Model file for the job. Use its own axes, mm. A direction names the side the tool comes from. Round coordinates to 2 decimals unless told otherwise and drop trailing zeros. Order: outer loops, then holes, each group sorted by start corner. A loop starts at its lowest first (then second) coordinate and runs counter-clockwise, first axis right, second up. Notation, with made-up numbers: (16.5, 23.5) -> (69.5, 23.5) arc R23 ccw to (69.5, 54.5) -> close; hole circle Ø9 at (25.5, 38.25). An arc over 180 degrees is marked (long way). Put each result on its own line as item: value. Start each with the question number.
Q1. Cut at C-C, the plane x = 27. List the corners of the cut face in (y, z) (3 decimals).
Q2. Flat gauge pins, fed straight in: P1, Ø10, axis at x = 20, y = 38.5, coming from the -Z side; P2, Ø7.5, axis at y = 7, z = -14, coming from the -X side; P3, Ø5, axis at x = 27, y = -4.5, coming from the +Z side (3 decimals). Where does each tip first touch, or does it go through?
Q3. Pull direction Z, two halves, no side cores. Call faces 1 (the face through (20, 8, -20)), 2 (the face through (21.035, 7.973, -10.515)), 3 (the face through (30, 68, -15)), 4 (the face through (13, 117, 15)): released by +Z, released by -Z, zero draft, split by the parting line, or undercut.
Q4. Cut at A-A, the plane y = 6.56. List the corners of the cut face in (x, z), and give its area (3 significant figures).
Q5. Cut at D-D, the plane z = -3.5. List the corners of the cut face in (x, y).
Q6. 3-axis set-ups, long thin cutter, end or side, ignore diameter. For faces 5 (the face through (25, -8, -8.025)), 6 (the face through (15, 44, -30)), 7 (the face through (10, 15, -4.95)): which of +Z, -Z, +X, -X, +Y, -Y reach the whole face in a straight line?
Q7. Cut at B-B, the plane z = -15. State how many separate pieces and enclosed holes the cut face has, and give its area (3 significant figures).
Q8. Probe L1, parallel to Z at x = 27.75, y = 23.56; L2, parallel to Y at x = 21, z = -15 (1 decimal); L3, parallel to X at y = 66.5, z = -0.5. List the from-to ranges inside material, lowest first.
Autodesk Inventor part; units mm, degrees
ref_plane "Work Plane1" through (0, 0, -15) normal (0, 0, 1) x (1, 0, 0)
ref_plane "YZ Plane" through (0, 0, 0) normal (1, 0, 0) x (0, 1, 0)
ref_plane "XZ Plane" through (0, 0, 0) normal (0, 1, 0) x (-1, 0, 0)
sketch "Sketch1" plane through (0, 0, 0) normal (0, 0, 1) x (1, 0, 0)
  line L0 (0, 0) -> (25, 0)
  line L1 (25, 0) -> (25, 40)
  line L2 (25, 40) -> (0, 40)
  line L3 (0, 40) -> (0, 0)
  dimension "d1" = 25
  dimension "d2" = 40
  dimension "d3" = 25
extrude "Extrusion1" add sketch "Sketch1" against normal blind 30
sketch "Sketch2" plane through (25, 0, 0) normal (1, 0, 0) x (0, 0, -1)
  line L0 (0, 0) -> (30, 0)
  circle A0 centre (15, 6.56) radius 2.46
extrude "Extrusion2" cut sketch "Sketch2" against normal blind 30
sketch "Sketch3" plane through (0, 0, 0) normal (-1, 0, 0) x (0, 0, 1)
  line L0 (0, 0) -> (-30, 0)
  line L1 (-25.05, 0) -> (-4.95, 0)
  line L2 (-4.95, 0) -> (-4.95, 33.12)
  line L3 (-4.95, 33.12) -> (-25.05, 33.12)
  line L4 (-25.05, 33.12) -> (-25.05, 0)
  dimension "d11" = 20.1
extrude "Extrusion3" cut sketch "Sketch3" against normal blind 20
sketch "Sketch4" plane through (0, 0, 0) normal (0, -1, 0) x (1, 0, 0)
  line L0 (20, -4.95) -> (20, -25.05)
  line L1 (20, -15) -> (25, -15)
  line L2 (25, 0) -> (25, -30)
  line L3 (20, -8.025) -> (25, -8.025)
  line L4 (25, -8.025) -> (25, -21.975)
  line L5 (25, -21.975) -> (20, -21.975)
  line L6 (20, -21.975) -> (20, -8.025)
  line L7 (20, -8.025) -> (25, -21.975) construction
  line L8 (25, -8.025) -> (20, -21.975) construction
  line L9 (25, -12.54) -> (25, -17.46)
  point P0 (0, 0)
  point P1 (22.5, -15)
  dimension "d14" = 13.95
extrude "Extrusion4" add sketch "Sketch4" along normal blind 15
sketch "Sketch5" plane through (20, 0, 0) normal (-1, 0, 0) x (0, 0, 1)
  circle A0 centre (-15, 6.56) radius 2.46
  circle A1 centre (-15, 6.56) radius 4.7025
  circle A2 centre (-15, 6.56) radius 2.46
  circle A3 centre (-15, 6.56) radius 2.46
  point P0 (0, 0)
  dimension "d17" = 9.405
extrude "Extrusion5" cut sketch "Sketch5" against normal blind 2.1
sketch "Sketch6" plane through (25, 0, 0) normal (1, 0, 0) x (0, 0, -1)
  circle A0 centre (15, 6.56) radius 4.7025
  line L0 (15, 6.56) -> (15, 23.56)
  circle A1 centre (15, 23.56) radius 2.46
  point P0 (0, 0)
  dimension "d20" = 17
  dimension "d21" = 4.92
extrude "Extrusion6" cut sketch "Sketch6" against normal blind 10 contours A1
sketch "Sketch7" plane through (20, 0, 0) normal (-1, 0, 0) x (0, 0, 1)
  circle A0 centre (-15, 23.56) radius 2.46
  circle A1 centre (-15, 23.56) radius 4.7025
  point P0 (0, 0)
  dimension "d24" = 9.405
extrude "Extrusion7" cut sketch "Sketch7" against normal blind 2.1
sketch "Sketch9" plane through (25, 0, 0) normal (1, 0, 0) x (0, 0, -1)
  circle A0 centre (15, 6.56) radius 2.46
  circle A1 centre (15, 6.56) radius 2.46
  circle A2 centre (15, 23.56) radius 2.46
  circle A3 centre (15, 23.56) radius 2.46
  line L0 (30, 40) -> (30, 0)
  line L1 (30, 0) -> (30, 40)
  line L2 (30, 40) -> (0, 40)
  line L3 (0, 40) -> (0, 0)
  line L4 (0, 0) -> (8.025, 0)
  line L5 (21.975, 0) -> (21.975, -15)
  line L6 (21.975, -15) -> (8.025, -15)
  line L7 (8.025, -15) -> (8.025, 0)
  line L8 (0, 0) -> (8.025, 0)
  line L9 (21.975, 0) -> (30, 0)
extrude "Extrusion8" add sketch "Sketch9" along normal blind 5
sketch "Sketch10" plane through (0, 40, 0) normal (0, 1, 0) x (1, 0, 0)
  line L0 (0, 30) -> (30, 30)
  line L1 (30, 0) -> (0, 0)
  line L2 (0, 30) -> (30, 30)
  line L3 (30, 30) -> (30, 0)
  line L4 (30, 0) -> (0, 0)
  line L5 (0, 0) -> (0, 30)
extrude "Extrusion9" add sketch "Sketch10" along normal blind 30
sketch "Sketch12" plane through (30, 0, 0) normal (1, 0, 0) x (0, 0, -1)
  circle A0 centre (15, 6.56) radius 2.46
  line L0 (15, 6.56) -> (15, 15.06)
  circle A1 centre (15, 15.06) radius 2.525
  point P0 (0, 0)
  dimension "d31" = 8.5
  dimension "d33" = 5.05
extrude "Extrusion10" cut sketch "Sketch12" against normal blind 30 contours A1
sketch "Sketch14" plane through (0, 0, 0) normal (0, 0, 1) x (1, 0, 0)
  line L0 (30, 70) -> (0, 70)
  line L1 (0, 70) -> (0, 100)
  line L2 (30, 0) -> (30, 70)
  line L3 (30, 122.5) -> (30, 70)
  line L4 (30, 105) -> (30, 100)
  line L5 (-12, 145) -> (15, 145)
  line L6 (-7, 142.5) -> (-12, 145)
  line L7 (-7, 102.5) -> (-12, 100)
  line L8 (-7, 102.5) -> (-2, 122.5)
  line L9 (-2, 122.5) -> (-7, 142.5)
  line L10 (30, 122.5) -> (15, 145)
  line L11 (0, 100) -> (-12, 100)
  point P0 (0, 0)
  dimension "d86" = 12
extrude "Extrusion12" add sketch "Sketch14" against normal blind 30
sketch "Sketch15" plane through (0, 0, -25.05) normal (-1, 0, 0) x (0, 0, 1)
  line L0 (0, 33.12) -> (20.1, 33.12)
  line L1 (20.1, 33.12) -> (20.1, 0)
  line L2 (0, 33.12) -> (20.1, 33.12)
  line L3 (20.1, 33.12) -> (20.1, 31.1)
  line L4 (20.1, 31.1) -> (0, 31.1)
  line L5 (0, 31.1) -> (0, 33.12)
  point P0 (25.05, 0)
  dimension "d57" = 2.02
extrude "Extrusion13" add sketch "Sketch15" against normal blind 20
sketch "Sketch24" plane through (0, 0, 0) normal (0, 0, 1) x (1, 0, 0)
  line L0 (0, 100) -> (-12, 100)
  line L1 (-12, 100) -> (-7, 102.5)
  line L2 (0, 100) -> (-12, 100)
  line L3 (-12, 100) -> (-7, 102.5)
  line L4 (-7, 102.5) -> (-2, 122.5)
  line L5 (-7, 102.5) -> (-2, 122.5)
  line L6 (-2, 122.5) -> (-7, 142.5)
  line L7 (-2, 122.5) -> (-7, 142.5)
  line L8 (-7, 142.5) -> (-12, 145)
  line L9 (-7, 142.5) -> (-12, 145)
  line L10 (-12, 145) -> (15, 145)
  line L11 (-12, 145) -> (15, 145)
  line L12 (15, 145) -> (30, 122.5)
  line L13 (15, 145) -> (30, 122.5)
  line L14 (30, 122.5) -> (30, 87.5)
  line L15 (30, 87.5) -> (0, 87.5)
  line L16 (0, 87.5) -> (0, 100)
  point P0 (0, 0)
  dimension "d87" = 35
  dimension "d88" = 30
extrude "Extrusion14" add sketch "Sketch24" along normal blind 15
ref_plane "Work Plane1" through (0, 0, -15) normal (0, 0, 1) x (1, 0, 0)
mirror "Mirror1" about plane through (0, 0, -15) normal (0, 0, 1) of "Extrusion14"
properties part number "rec_b_40mm_x_60mm"
Ans:
1. outline: (-15, -21.975) -> (0, -21.975) -> (0, -30) -> (87.5, -30) -> (87.5, -45) -> (127, -45) -> (127, 15) -> (87.5, 15) -> (87.5, 0) -> (0, 0) -> (0, -8.025) -> (-15, -8.025) -> close; hole circle Ø4.92 at (6.56, -15); hole circle Ø5.05 at (15.06, -15); hole circle Ø4.92 at (23.56, -15)
2. P1: stops at z = -30
2. P2: stops at x = 20
2. P3: stops at z = -8.025
3. face 1: undercut
3. face 2: undercut
3. face 3: zero draft
3. face 4: released by +Z
4. outline: (0, -30) -> (30, -30) -> (30, -17.46) -> (22.1, -17.46) -> (22.1, -19.7) -> (20, -19.7) -> (20, -25.05) -> (0, -25.05) -> close; (0, -4.95) -> (20, -4.95) -> (20, -10.3) -> (22.1, -10.3) -> (22.1, -12.54) -> (30, -12.54) -> (30, 0) -> (0, 0) -> close
4. area: 439 mm^2
5. outline: (-12, 100) -> (0, 100) -> (0, 0) -> (30, 0) -> (30, 122.5) -> (15, 145) -> (-12, 145) -> (-7, 142.5) -> (-2, 122.5) -> (-7, 102.5) -> close
6. face 5: +Z, +X, -X, -Y
6. face 6: -Z, +X, -X, -Y
6. face 7: -X, -Y
7. separate pieces: 4
7. enclosed holes: 0
7. area: 3,770 mm^2
8. L1: z = -30 to -17.46, -12.54 to 0
8. L2: y = -15 to 1.9, 11.3 to 12.5, 17.6 to 18.9, 28.3 to 136
8. L3: x = 0 to 30
